Part print with two shaded views. Sizes in mm from the minimum x, y, z corner. Coordinates: 2 decimals unless noted, no trailing zeros. Order: outer loops, then holes, each group sorted by start corner. A loop starts at its lowest first (then second) coordinate and runs counter-clockwise, first axis right, second up. Notation, with made-up numbers: M 34,-9.75 L 80,-9.75 A19 ccw 80,3.25 Z; hole C 63,11 d2. An arc over 180 degrees is marked long. Answer in a Markdown table with one row per item. Add a question column.
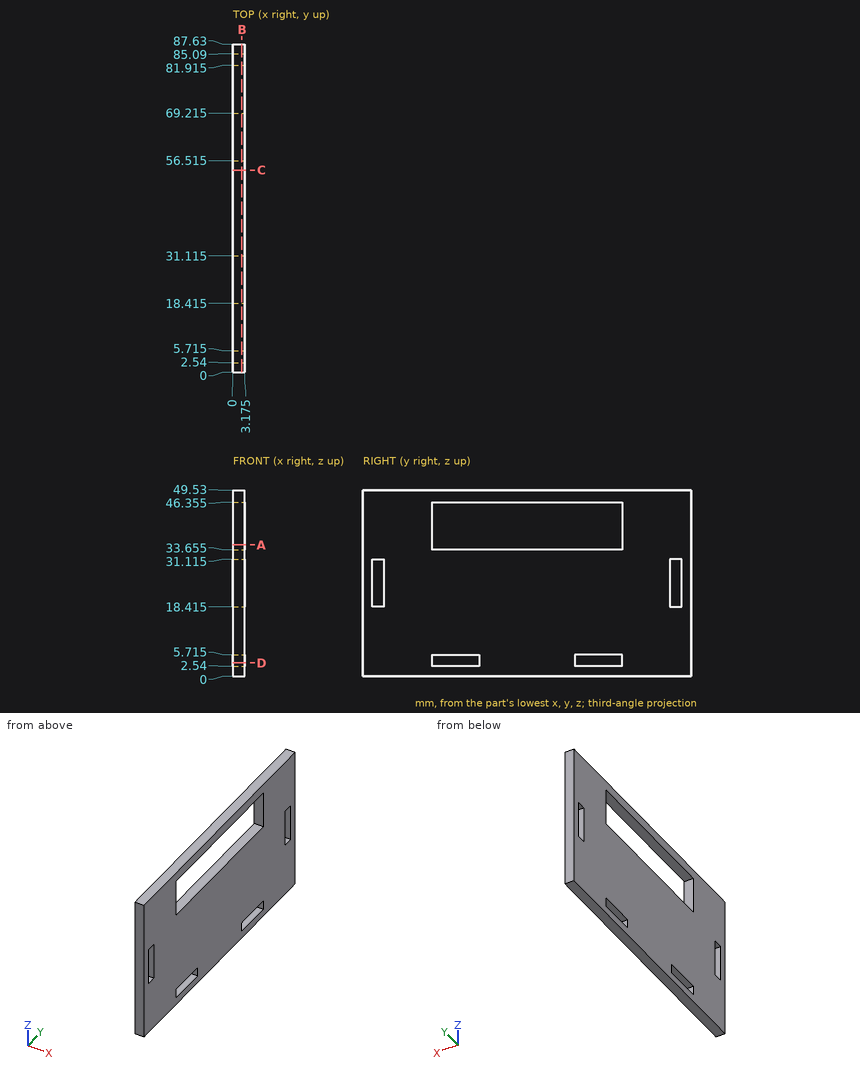
(1) Slice it at A-A (z = 35). List the corners of the cut face in (x, y) (3 decimals), and give its area (3 significant figures).
(2) Wall check: line 1 (Z direction, x = 2.25, y = 20) (3 decimals); line 2 (Y direction, x = 0.9, z = 3) (3 decimals); line 3 (Y direction, x = 0.3, z = 42) (3 decimals). Give the ranges that are in metal, low to high.
(3) Slice it at B-B (x = 2.4). List the corners of the cut face in (y, z) (3 decimals).
(4) Slice it at C-C (y = 54). List the corners of the cut face in (x, z) (3 decimals).
(5) Slice it at D-D (z = 3.5). List the corners of the cut face in (x, y) (3 decimals).
Computed:
| question | item | result |
|---|---|---|
| 1 | outline | M 0,0 L 3.175,0 L 3.175,18.415 L 0,18.415 Z; M 0,69.215 L 3.175,69.215 L 3.175,87.63 L 0,87.63 Z |
| 1 | area | 117 mm^2 |
| 2 | line 1 | z = 0 to 2.54, 5.715 to 33.655, 46.355 to 49.53 |
| 2 | line 2 | y = 0 to 18.415, 31.115 to 56.515, 69.215 to 87.63 |
| 2 | line 3 | y = 0 to 18.415, 69.215 to 87.63 |
| 3 | outline | M 0,0 L 87.63,0 L 87.63,49.53 L 0,49.53 Z; hole M 2.54,18.415 L 5.715,18.415 L 5.715,31.115 L 2.54,31.115 Z; hole M 18.415,2.54 L 31.115,2.54 L 31.115,5.715 L 18.415,5.715 Z; hole M 18.415,33.655 L 69.215,33.655 L 69.215,46.355 L 18.415,46.355 Z; hole M 56.515,2.54 L 69.215,2.54 L 69.215,5.715 L 56.515,5.715 Z; hole M 81.915,18.415 L 85.09,18.415 L 85.09,31.115 L 81.915,31.115 Z |
| 4 | outline | M 0,0 L 3.175,0 L 3.175,33.655 L 0,33.655 Z; M 0,46.355 L 3.175,46.355 L 3.175,49.53 L 0,49.53 Z |
| 5 | outline | M 0,0 L 3.175,0 L 3.175,18.415 L 0,18.415 Z; M 0,31.115 L 3.175,31.115 L 3.175,56.515 L 0,56.515 Z; M 0,69.215 L 3.175,69.215 L 3.175,87.63 L 0,87.63 Z |
